```python
from build123d import *

# Parameters (mm, degrees)
EXTRUDE_1_DEPTH          = 6
PATTERN_CIRCULAR_1_COUNT = 16


with BuildPart() as part:
    # Эскиз2 → Бобышка-Вытянуть1 (new body)
    with BuildSketch(Plane.XY):
        with BuildLine():
            Line((0, 0), (0, 28.194026186))
            ThreePointArc((0, 28.194026186), (2.762782753, 29.182565662), (4.271319896, 31.699407834))
            ThreePointArc((4.271319896, 31.699407834), (5.166850576, 34.134348257), (6.766906166, 36.176585307))
            ThreePointArc((6.766906166, 36.176585307), (7.18010932, 36.096847143), (7.592373731, 36.012389599))
            ThreePointArc((7.592373731, 36.012389599), (8.289102058, 33.513293823), (8.184653165, 30.920997449))
            ThreePointArc((8.184653165, 30.920997449), (8.615205955, 28.018446308), (10.789386713, 26.047883733))
            Line((10.789386713, 26.047883733), (0, 0))
        make_face()
    extrude_1 = extrude(amount=EXTRUDE_1_DEPTH)

    # Круговой массив1: Бобышка-Вытянуть1 ×16 about axis
    pattern_circular_1_axis = Axis((0, 0, 0), (0, 0, 1))
    for i in range(1, PATTERN_CIRCULAR_1_COUNT):
        add(extrude_1.rotate(pattern_circular_1_axis, i * 360 / PATTERN_CIRCULAR_1_COUNT))


solid = part.part
```
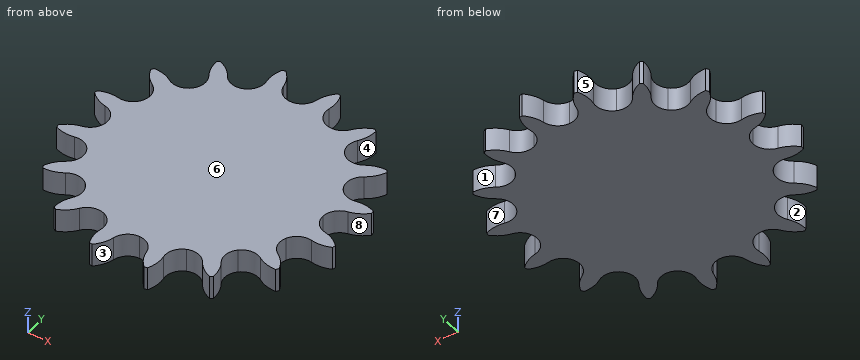
Model file for the job. Use its own axes, mm. Face numbers are marked on the shaded views. A direction names the side the tool comes from. Give positions to 0.01 mm unless a question says otherwise; leave off trailing zeros. Loops run counter-clockwise (first coordinate to the right, second up) from the corner with the lowest first, then second, coordinate; pieces in that order, holes last. Notation, with made-up numbers: (-16.5, -1.5) -> (-8.5, -1.5) arc R30 cw to (-8.5, 28.5) -> close; hole circle Ø6 at (-36, -30.75). An arc over 180 degrees is marked (long way). Use CSV: the item, a comma, the result in double quotes. Start each with the question number.
1) Slice it at B-B on x = 13.5. Give the cut face in (y, z).
2) Slice it at A-A on y = -22. Give the cut face in (x, z), plus the area to 3 significant figures.
3) Tool access for the marked faces 1, 2, 3 and 4: list every direction of +Z, -Z, +X, -X, +Y, -Y with a clear straight run to the whole face (end or side of a thin tool).
4) Wall check: line 1 (Y direction, x = 29.5, z = 4.4); line 2 (Y direction, x = 29, z = 3.15); line 3 (Y direction, x = 27.5, z = 5). Give the ranges that are in metal, low to high.
5) Flat gauge pins, fed straight in: pin 1 Ø2 at (x, z) = (-15, 2.5) entering from +Y; pin 2 Ø1.5 at (y, z) = (3, 2) entering from +X; pin 3 Ø1 at (y, z) = (24, 4) entering from +X. Where does each tip first touch, or does it go through?
6) Mould opens along X. For the marked faces 5, 6, 7 and 8 say: released by +X, released by -X, zero draft, split by the parting line, or undercut.
Computed values:
1,outline,"(-25.84, 0) -> (25.84, 0) -> (25.84, 6) -> (-25.84, 6) -> close"
2,outline,"(-18.78, 0) -> (18.78, 0) -> (18.78, 6) -> (-18.78, 6) -> close"
2,area,"225 mm^2"
3,face 1,"+Z, -Z, +Y"
3,face 2,"+Z, -Z, -X"
3,face 3,"+Z, -Z, -Y"
3,face 4,"+Z, -Z, +X"
4,line 1,"y = -20.78 to -17.76, -8.14 to -3.11, 3.11 to 8.14, 17.76 to 20.78"
4,line 2,"y = -20.73 to -17.2, -8.23 to -2.52, 2.52 to 8.23, 17.2 to 20.73"
4,line 3,"y = -20.39 to -15.97, -8.94 to 8.94, 15.97 to 20.39"
5,pin 1,"stops at y = 27.54"
5,pin 2,"stops at x = 30.33"
5,pin 3,"stops at x = 18.92"
6,face 5,"released by -X"
6,face 6,"zero draft"
6,face 7,"undercut"
6,face 8,"released by +X"
